```python
from build123d import *

# Parameters (mm, degrees)
SKETCH1_R           = 7.5
BOSS_EXTRUDE1_DEPTH = 2.5


with BuildPart() as part:
    # Sketch1 → Boss-Extrude1 (new, symmetric)
    with BuildSketch(Plane(origin=(0, 0, 0), x_dir=(0, 0, -1), z_dir=(1, 0, 0))):
        Polygon((100, -25), (100, 25), (90, 25), (-90, 40), (-100, 40), (-100, -40), (-90, -40), (90, -25), align=None)
        Circle(SKETCH1_R, mode=Mode.SUBTRACT)
        with Locations((-60, 0)):
            Circle(SKETCH1_R, mode=Mode.SUBTRACT)
        with Locations((60, 0)):
            Circle(SKETCH1_R, mode=Mode.SUBTRACT)
    extrude(amount=BOSS_EXTRUDE1_DEPTH, both=True)


solid = part.part
```
The listing builds one solid part. Answer for the finished solid, in the listing's coordinates (mm). A direction names the side the tool comes from. Round coordinates to 2 decimals unless told otherwise and drop trailing zeros. Write each loop counter-clockwise with the first axis right and the second up, starting at its lowest first coordinate (ties: lowest second). Pieces come first, ordered by that corner, then holes. Notation, with made-up numbers: (83, 9.25) -> (129, 9.25) arc R20 ccw to (129, 29.25) -> close; hole circle Ø8 at (-13, -19.75). An arc over 180 degrees is marked (long way). Answer as a JSON object with one key per item and string values. Group by question number.
Q1. Section A-A (z = 60) is taken. Write down the section's boundary in (x, y), plus the area to 3 significant figures.
Q2. Each of these flat-tipped pins is pushed along its axis until it touches: pin 1 Ø2.5 at (x, z) = (1, -96.5) entering from +Y; pin 2 Ø24 at (y, z) = (0, 60) entering from +X; pin 3 Ø12 at (y, z) = (0, 0) entering from +X. Where does it stop, or does it pass through?
Q3. Section B-B (y = 0) is taken. Write down the section's boundary in (x, z), plus the area to 3 significant figures.
Q4. Section D-D (z = -60) is taken. Write down the section's boundary in (x, y).
Q5. Straight lines are drawn through the part: line 1 along Z through (x, y) = (0.7, 5); line 2 along Y through (x, z) = (1.5, 60); line 3 along Y through (x, z) = (-1.5, -60). For each, find the intervals that lie inside material, in ascending order.
Q6. Section C-C (x = 0) is taken. Write down the section's boundary in (y, z), plus the area to 3 significant figures.
Q7. Determine the mould class of faces 4 (the face through (0, -40, 95)), 5 (the face through (0, 40, 95)), 6 (the face through (-0.035, 0.33, 67.493)) for opening direction Y: pulls with the +Y half, pulls with the -Y half, needs draft (parallel to the pull), parting line crosses it, or undercut.
Q8. Which of the six approach directions +Z, -Z, +X, -X, +Y, -Y give full straight-line access (tool end or side, diameter ignored) to faces 1 (the face through (0, -25, -95)), 2 (the face through (0, 25, -95)), 3 (the face through (2.5, 1, 24))?
Check values:
{
 "1": {"outline": "(-2.5, -37.5) -> (2.5, -37.5) -> (2.5, -7.5) -> (-2.5, -7.5) -> close; (-2.5, 7.5) -> (2.5, 7.5) -> (2.5, 37.5) -> (-2.5, 37.5) -> close", "area": "300 mm^2"},
 "2": {"pin 1": "y = 25", "pin 2": "x = 2.5", "pin 3": "through"},
 "3": {"outline": "(-2.5, -100) -> (2.5, -100) -> (2.5, -67.5) -> (-2.5, -67.5) -> close; (-2.5, -52.5) -> (2.5, -52.5) -> (2.5, -7.5) -> (-2.5, -7.5) -> close; (-2.5, 7.5) -> (2.5, 7.5) -> (2.5, 52.5) -> (-2.5, 52.5) -> close; (-2.5, 67.5) -> (2.5, 67.5) -> (2.5, 100) -> (-2.5, 100) -> close", "area": "775 mm^2"},
 "4": {"outline": "(-2.5, -27.5) -> (2.5, -27.5) -> (2.5, -7.5) -> (-2.5, -7.5) -> close; (-2.5, 7.5) -> (2.5, 7.5) -> (2.5, 27.5) -> (-2.5, 27.5) -> close"},
 "5": {"line 1": "-100 to -65.59, -54.41 to -5.59, 5.59 to 54.41, 65.59 to 100", "line 2": "-37.5 to -7.5, 7.5 to 37.5", "line 3": "-27.5 to -7.5, 7.5 to 27.5"},
 "6": {"outline": "(-40, 90) -> (-25, -90) -> (-25, -100) -> (25, -100) -> (25, -90) -> (40, 90) -> (40, 100) -> (-40, 100) -> close; hole circle Ø15 at (0, -60); hole circle Ø15 at (0, 0); hole circle Ø15 at (0, 60)", "area": "12,500 mm^2"},
 "7": {"face 4": "pulls with the -Y half", "face 5": "pulls with the +Y half", "face 6": "undercut"},
 "8": {"face 1": "-Z, +X, -X, -Y", "face 2": "-Z, +X, -X, +Y", "face 3": "+Z, -Z, +X, +Y, -Y"}
}
